Verification items for the finished model (mm, model axes). Face numbers are marked on the shaded views. Round coordinates to 2 decimals unless told otherwise and drop trailing zeros. Loops run counter-clockwise (first coordinate to the right, second up) from the corner with the lowest first, then second, coordinate; pieces in that order, holes last. Notation, with made-up numbers: (55.25, -26.75) -> (78.25, -26.75) arc R30 cw to (78.25, 8.25) -> close; hole circle Ø3 at (5, 86). An arc over 180 degrees is marked (long way). Use CSV: the item, a comma, the result in double quotes. Start each with the question number.
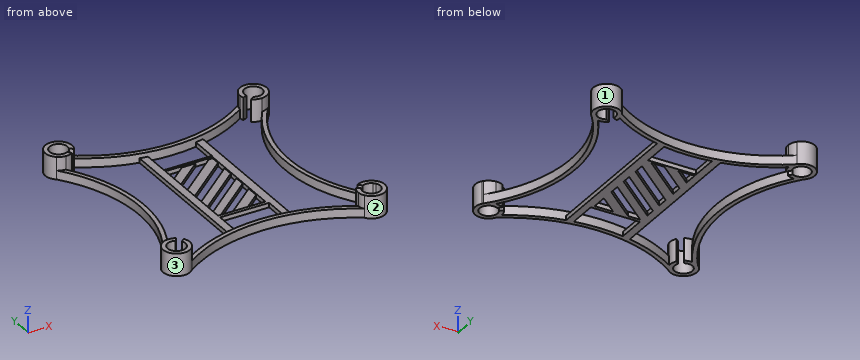
```python
from build123d import *

# Parameters (mm, degrees)
F1_DEPTH = 10
F2_DEPTH = 4
F4_DEPTH = 2
F5_W     = 21.1815265939
F5_H     = 39.6702438593
F6_DEPTH = 0.5
F8_DEPTH = 1.501


with BuildPart() as f1:
    # F0 (on Top) → F1 (new body)
    with BuildSketch(Plane.XY):
        with BuildLine():
            Line((-62.1572475363, -49.3555771993), (-60.9726684437, -47.7181399205))
            ThreePointArc((-60.9726684437, -47.7181399205), (-62.5677534438, -47.1070816307), (-64.2703892861, -46.970262115))
            ThreePointArc((-64.2703892861, -46.970262115), (-66.055157525, -47.2638248655), (-67.5855421771, -48.2279304467))
            ThreePointArc((-67.5855421771, -48.2279304467), (-68.2915955562, -57.0411338211), (-59.4503077741, -56.9892161196))
            ThreePointArc((-59.4503077741, -56.9892161196), (-58.503657354, -55.3744867929), (-57.9284491894, -53.593298037))
            ThreePointArc((-57.9284491894, -53.593298037), (-58.0525320787, -51.5916655896), (-58.8293116163, -49.7427354752))
            Line((-58.8293116163, -49.7427354752), (-60.3885015243, -51.0333806943))
            ThreePointArc((-60.3885015243, -51.0333806943), (-66.6476098165, -55.8605427209), (-62.1572475363, -49.3555771993))
        make_face()
    extrude(amount=F1_DEPTH)



with BuildPart() as f1b:
    # F0 (on Top) → F1, piece 2 (new body)
    with BuildSketch(Plane.XY):
        with BuildLine():
            ThreePointArc((17.1087630149, -53.4675772739), (17.3345654758, -55.024615232), (18.0236412267, -56.4390156575))
            ThreePointArc((18.0236412267, -56.4390156575), (26.3870023747, -58.2706581148), (28.0672567096, -49.8755721025))
            ThreePointArc((28.0672567096, -49.8755721025), (27.8342119425, -49.6100285483), (27.6026930798, -49.343153561))
            ThreePointArc((27.6026930798, -49.343153561), (25.6605798387, -47.9272938937), (23.3536224131, -47.2531945869))
            ThreePointArc((23.3536224131, -47.2531945869), (21.5502161664, -47.4529085878), (19.8889698394, -48.1825800302))
            Line((19.8889698394, -48.1825800302), (21.3739898723, -49.6418572585))
            ThreePointArc((21.3739898723, -49.6418572585), (23.6329189205, -49.2830550049), (25.7191516005, -50.2206757743))
            ThreePointArc((25.7191516005, -50.2206757743), (26.0985339145, -50.66438117), (26.4819704741, -51.1045877386))
            ThreePointArc((26.4819704741, -51.1045877386), (23.0622875716, -57.2478053636), (19.7737803157, -51.0333806943))
            Line((19.7737803157, -51.0333806943), (17.9670109528, -50.1490486996))
            ThreePointArc((17.9670109528, -50.1490486996), (17.2958667801, -51.7457209867), (17.1087630149, -53.4675772739))
        make_face()
    extrude(amount=F1_DEPTH)


with BuildPart() as f1c:
    # F0 (on Top) → F1, piece 3 (new body)
    with BuildSketch(Plane.XY):
        with BuildLine():
            ThreePointArc((26.0956428667, 29.3550487731), (25.6609988664, 38.5030065298), (16.7099807908, 36.5656573261))
            ThreePointArc((16.7099807908, 36.5656573261), (16.1402416091, 35.1660163707), (16.0062342849, 33.6608122064))
            ThreePointArc((16.0062342849, 33.6608122064), (16.109517209, 32.6334069675), (16.3874284639, 31.6389250815))
            Line((16.3874284639, 31.6389250815), (18.1665952148, 32.6217676343))
            ThreePointArc((18.1665952148, 32.6217676343), (22.4683173599, 37.7181778333), (25.4838572425, 31.7696713362))
            ThreePointArc((25.4838572425, 31.7696713362), (23.0337650915, 29.879413145), (19.9683402486, 30.3027311227))
            Line((19.9683402486, 30.3027311227), (18.2454213302, 29.0694802814))
            ThreePointArc((18.2454213302, 29.0694802814), (20.1934444417, 28.0252417902), (22.3873843451, 27.7571825242))
            ThreePointArc((22.3873843451, 27.7571825242), (24.3427437086, 28.3211852273), (26.0956428667, 29.3550487731))
        make_face()
    extrude(amount=F1_DEPTH)


with BuildPart() as f1d:
    # F0 (on Top) → F1, piece 4 (new body)
    with BuildSketch(Plane.XY):
        with BuildLine():
            ThreePointArc((-68.732125287, 29.3414321402), (-67.1003065349, 28.443679964), (-65.2817843614, 28.0414753968))
            ThreePointArc((-65.2817843614, 28.0414753968), (-63.5823726874, 28.2029549498), (-61.9972172476, 28.8364830984))
            Line((-61.9972172476, 28.8364830984), (-63.1768257939, 30.471091811))
            ThreePointArc((-63.1768257939, 30.471091811), (-67.9311262024, 36.7498087051), (-61.2988677278, 32.5025971803))
            Line((-61.2988677278, 32.5025971803), (-59.7430924035, 31.1312410763))
            ThreePointArc((-59.7430924035, 31.1312410763), (-59.1314611672, 32.7570252654), (-59.0111762545, 34.4898837532))
            ThreePointArc((-59.0111762545, 34.4898837532), (-59.5181526175, 36.4535488342), (-60.6284022775, 38.1507086015))
            ThreePointArc((-60.6284022775, 38.1507086015), (-69.4096636596, 38.09668268), (-68.732125287, 29.3414321402))
        make_face()
    extrude(amount=F1_DEPTH)


with BuildPart() as f1_1:
    add(f1.part)

    add(f1b.part)  # F2 merges F1b

    add(f1c.part)  # F2 merges F1c

    add(f1d.part)  # F2 merges F1d
    # F0 (on Top) → F2 (join)
    with BuildSketch(Plane.XY):
        with BuildLine():
            ThreePointArc((-67.5855421771, -48.2279304467), (-66.055157525, -47.2638248655), (-64.2703892861, -46.970262115))
            ThreePointArc((-64.2703892861, -46.970262115), (-53.1706504597, -9.3079154321), (-65.2817843614, 28.0414753968))
            ThreePointArc((-65.2817843614, 28.0414753968), (-67.1003065349, 28.443679964), (-68.732125287, 29.3414321402))
            ThreePointArc((-68.732125287, 29.3414321402), (-55.1716501295, -9.251280509), (-67.5855421771, -48.2279304467))
        make_face()
        with BuildLine():
            ThreePointArc((16.7099807908, 36.5656573261), (-22.2207470412, 24.5972113145), (-60.6284022775, 38.1507086015))
            ThreePointArc((-60.6284022775, 38.1507086015), (-59.5181526175, 36.4535488342), (-59.0111762545, 34.4898837532))
            ThreePointArc((-59.0111762545, 34.4898837532), (-21.6294297382, 22.5876579696), (16.0062342849, 33.6608122064))
            ThreePointArc((16.0062342849, 33.6608122064), (16.1402416091, 35.1660163707), (16.7099807908, 36.5656573261))
        make_face()
        with BuildLine():
            ThreePointArc((27.6026930798, -49.343153561), (12.6512102924, -10.2659396101), (26.0956428667, 29.3550487731))
            ThreePointArc((26.0956428667, 29.3550487731), (24.3427437086, 28.3211852273), (22.3873843451, 27.7571825242))
            ThreePointArc((22.3873843451, 27.7571825242), (10.6432367974, -9.9055102447), (23.3536224131, -47.2531945869))
            ThreePointArc((23.3536224131, -47.2531945869), (25.6605798387, -47.9272938937), (27.6026930798, -49.343153561))
        make_face()
        with BuildLine():
            ThreePointArc((-57.9284491894, -53.593298037), (-58.503657354, -55.3744867929), (-59.4503077741, -56.9892161196))
            ThreePointArc((-59.4503077741, -56.9892161196), (-20.798072436, -44.7819602715), (18.0236412267, -56.4390156575))
            ThreePointArc((18.0236412267, -56.4390156575), (17.3345654758, -55.024615232), (17.1087630149, -53.4675772739))
            ThreePointArc((17.1087630149, -53.4675772739), (-20.4278543179, -42.780323647), (-57.9284491894, -53.593298037))
        make_face()
    extrude(amount=F2_DEPTH)

    # F3 (on face) → F4 (join)
    with BuildSketch(Plane(origin=(0, 0, 0), x_dir=(1, 0, 0), z_dir=(0, 0, -1))):
        with BuildLine():
            Line((-9.3221692368, 30.8540649712), (-31.277757138, 30.8540649712))
            Line((-31.277757138, 30.8540649712), (-31.277757138, 43.6344668102))
            ThreePointArc((-31.277757138, 43.6344668102), (-33.0149879746, 43.9288902719), (-34.7443595529, 44.266425601))
            Line((-34.7443595529, 44.266425601), (-34.7443595529, 30.8540649712))
            Line((-34.7443595529, 30.8540649712), (-34.7443595529, -11.383831501))
            Line((-34.7443595529, -11.383831501), (-34.7443595529, -24.0321703309))
            ThreePointArc((-34.7443595529, -24.0321703309), (-33.0152564459, -23.6903099606), (-31.277757138, -23.3940630665))
            Line((-31.277757138, -23.3940630665), (-31.277757138, -11.383831501))
            Line((-31.277757138, -11.383831501), (-9.8225176334, -11.383831501))
            Line((-9.8225176334, -11.383831501), (-9.8225176334, -23.5040877089))
            ThreePointArc((-9.8225176334, -23.5040877089), (-8.027086971, -23.8300565225), (-6.2412018888, -24.2048116485))
            Line((-6.2412018888, -24.2048116485), (-6.2412018888, -11.383831501))
            Line((-6.2412018888, -11.383831501), (-6.2412018888, 30.8540649712))
            Line((-6.2412018888, 30.8540649712), (-6.2412018888, 44.1910067814))
            ThreePointArc((-6.2412018888, 44.1910067814), (-7.7786273027, 43.8971600473), (-9.3221692368, 43.6373503013))
            Line((-9.3221692368, 43.6373503013), (-9.3221692368, 30.8540649712))
        make_face()
    extrude(amount=-F4_DEPTH)

    # F5 (on face) → F6 (cut)
    with BuildSketch(Plane.XY.offset(2)):
        with Locations((-20.6869938411, -9.4783511013)):
            Rectangle(F5_W, F5_H)
    extrude(amount=-F6_DEPTH, mode=Mode.SUBTRACT)

    # F7 (on face) → F8 (cut, through all)
    with BuildSketch(Plane.XY.offset(1.5)):
        Polygon((-31.277757138, 10.3567708284), (-31.277757138, 4.1535533965), (-23.8866638392, 10.3567708284), align=None)
        Polygon((-17.7311521972, 10.3567708284), (-31.277757138, -1.0126616107), (-31.277757138, -5.9374999255), (-11.8632393173, 10.3567708284), align=None)
        Polygon((-10.0962305441, 6.3696975482), (-31.277757138, -11.4075932652), (-31.277757138, -16.3320098072), (-10.0962305441, 1.4452810061), align=None)
        Polygon((-10.0962305441, -3.244678803), (-31.277757138, -21.0219696164), (-31.277757138, -25.2428706735), (-10.0962305441, -7.4655798602), align=None)
        Polygon((-10.0962305441, -16.7659351889), (-10.0962305441, -12.173710581), (-30.5181462318, -29.3134730309), (-25.0465404242, -29.3134730309), align=None)
        Polygon((-10.0962305441, -29.3134730309), (-10.0962305441, -22.3181112129), (-18.4311587363, -29.3134730309), align=None)
    extrude(amount=-F8_DEPTH, mode=Mode.SUBTRACT)


solid = f1_1.part
```
Q1. Depth check by flat-ended pin: pin 1 Ø12 at (x, y) = (-49, -15.5) entering from +Z; pin 2 Ø0.6 at (y, z) = (16, 0.5) entering from -X; pin 3 Ø17 at (x, y) = (-25, -9.5) entering from +Z; pin 4 Ø4 at (x, y) = (-13.5, -49) entering from -Z. Enter the tip coordinate at first touch or a pass-through.
Q2. Thickness scan on L1, parallel to X at y = 33.5, z = 5.25; L2, parallel to Y at x = 22, z = 7.75; L3, parallel to Y at x = -61.5, z = 4.25. Record the ranges inside material, lowest first. Write a range as from..to.
Q3. Cross-section at D-D (x = -48). Record the boundary of the cut face in (y, z).
Q4. Cross-section at C-C (y = -41.5). Record the boundary of the cut face in (x, z), and give its area (3 significant figures).
Q5. Release check for a two-part mould opening along Y. For the marked faces 1, 2 and 3 record: +Y half, -Y half, draft (parallel to the pull), parting line (faces both ways), or undercut.
Q6. Cross-section at B-B (x = -27.5). State how many separate pieces and enclosed holes the cut face has, and give its area (3 significant figures).
Q7. Cross-section at A-A (y = -18.5). Record the boundary of the cut face in (x, z).
Answer list:
1,pin 1,"stops at z = 4"
1,pin 2,"stops at x = -60.87"
1,pin 3,"stops at z = 2"
1,pin 4,"passes through"
2,L1,"x = -70.97..-68.96, -61.03..-59.02, 16.01..18.01, 26..28"
2,L2,"y = -59.15..-57.09, -49.4..-47.35, 27.75..29.75, 37.75..39.75"
2,L3,"y = -58.46..-56.16, -48.45..-47.46, 35.98..38.91"
3,outline,"(-50.59, 0) -> (-48.42, 0) -> (-48.42, 4) -> (-50.59, 4) -> close; (28.32, 0) -> (30.51, 0) -> (30.51, 4) -> (28.32, 4) -> close"
4,outline,"(-63.28, 0) -> (-61, 0) -> (-61, 4) -> (-63.28, 4) -> close; (-34.74, 0) -> (-31.28, 0) -> (-31.28, 2) -> (-34.74, 2) -> close; (-9.32, 0) -> (-6.24, 0) -> (-6.24, 2) -> (-9.32, 2) -> close; (19.51, 0) -> (21.85, 0) -> (21.85, 4) -> (19.51, 4) -> close"
4,area,"31.6 mm2"
5,face 1,"undercut"
5,face 2,"parting line"
5,face 3,"undercut"
6,separate pieces,"8"
6,enclosed holes,"0"
6,area,"51.3 mm2"
7,outline,"(-55.7, 0) -> (-53.68, 0) -> (-53.68, 4) -> (-55.7, 4) -> close; (-34.74, 0) -> (-28.27, 0) -> (-28.27, 1.5) -> (-31.28, 1.5) -> (-31.28, 2) -> (-34.74, 2) -> close; (-23.24, 0) -> (-17.63, 0) -> (-17.63, 1.5) -> (-23.24, 1.5) -> close; (-12.16, 0) -> (-6.24, 0) -> (-6.24, 2) -> (-10.1, 2) -> (-10.1, 1.5) -> (-12.16, 1.5) -> close; (11.34, 0) -> (13.36, 0) -> (13.36, 4) -> (11.34, 4) -> close"
